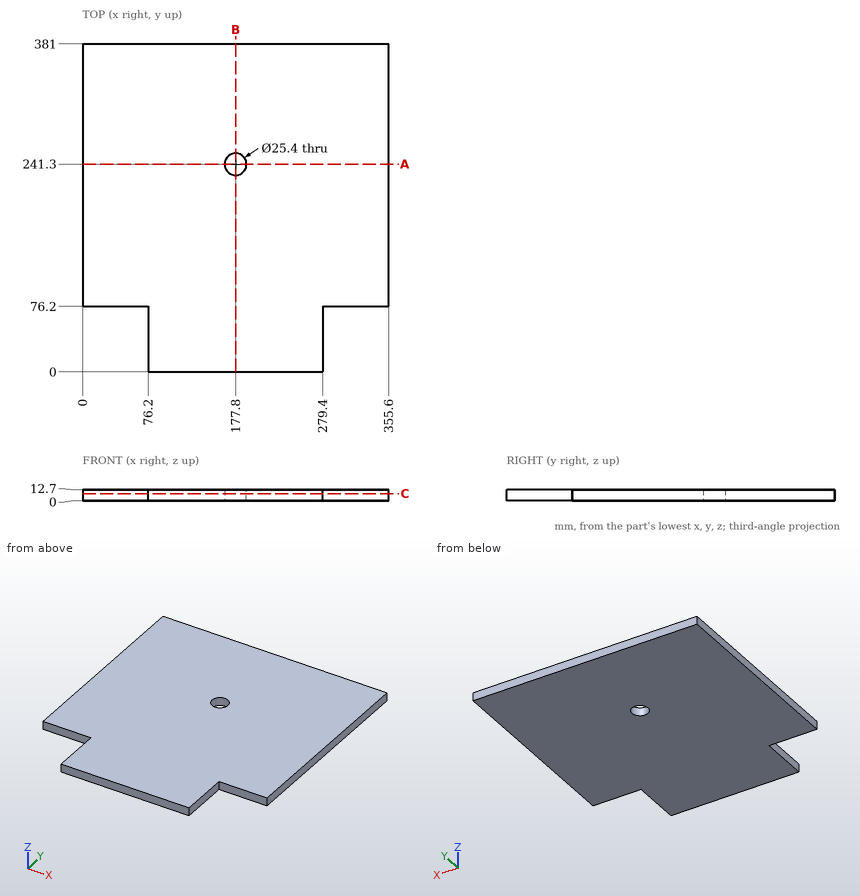
Verification items for this drawing (mm, ordinates from the low corner). Round coordinates to 2 decimals unless told otherwise and drop trailing zeros. Order: outer loops, then holes, each group sorted by start corner. A loop starts at its lowest first (then second) coordinate and runs counter-clockwise, first axis right, second up.
1) Cross-section at C-C, the plane z = 8.5. Record the cut outline in (x, y), plus the area to 3 significant figures.
Geometry says:
outline: (0, 76.2) - (76.2, 76.2) - (76.2, 0) - (279.4, 0) - (279.4, 76.2) - (355.6, 76.2) - (355.6, 381) - (0, 381) - close; hole circle Ø25.4 at (177.8, 241.3)
area: 123,000 mm2
2) Material ranges on line 1 (Y direction, x = 177.8, z = 7.25); line 2 (X direction, y = 241.3, z = 5.25); line 3 (Y direction, x = 324, z = 7), recorded low to high.
Geometry says:
line 1: y = 0 to 228.6, 254 to 381
line 2: x = 0 to 165.1, 190.5 to 355.6
line 3: y = 76.2 to 381
3) Cross-section at B-B, the plane x = 177.8. Record the cut outline in (y, z).
Geometry says:
outline: (0, 0) - (228.6, 0) - (228.6, 12.7) - (0, 12.7) - close; (254, 0) - (381, 0) - (381, 12.7) - (254, 12.7) - close
4) Depth check by flat-ended pin: pin 1 (6.5 mm diameter, centred on y = 31, z = 5, fed in from +X); pin 2 (6.5 mm diameter, centred on x = 319, z = 4, fed in from -Y). Enter the tip coordinate at first touch or a pass-through.
Geometry says:
pin 1: stops at x = 279.4
pin 2: stops at y = 76.2
5) Cross-section at A-A, the plane y = 241.3. Record the cut outline in (x, z).
Geometry says:
outline: (0, 0) - (165.1, 0) - (165.1, 12.7) - (0, 12.7) - close; (190.5, 0) - (355.6, 0) - (355.6, 12.7) - (190.5, 12.7) - close
